Input: dimensioned drawing with shaded views. Units: mm. Origin: part minimum x, y, z. A direction names the side the tool comes from. Give positions to 0.01 mm unless a question says otherwise; leave off trailing zeros. Loops run counter-clockwise (first coordinate to the right, second up) from the corner with the lowest first, then second, coordinate; pieces in that order, holes last. Notation, with made-up numbers: M 53,10.5 L 93,10.5 A21 ccw 93,41.5 Z; hole C 37.5,69.25 d10. An arc over 180 degrees is marked long. Use CSV: the item, a comma, the result in double quotes. Start each with the question number.
Q1. Pull-direction query (X, two-part tool) for the marked faces 3, 4 and 5; classes: released by +X, released by -X, zero draft, split by the parting line, or undercut.
Q2. Section D-D, the plane z = 19. Output: boundary loops of the cut face in (x, y), plus the area to 3 significant figures.
Q3. Reachability of the marked faces 1 and 2 from +Z, -Z, +X, -X, +Y, -Y: full face, straight path, thin tool, end or side. Return the list, or none.
Q4. Material intervals for line 1 along X through (y, z) = (5.75, 48.5) (1 decimal); line 2 along X through (y, z) = (0.75, 27.5); line 3 along Z through (x, y) = (49.75, 4), sorted ascending.
Q5. Section A-A, the plane z = 27.25. Output: boundary loops of the cut face in (x, y), plus the area to 3 significant figures.
Q6. Section B-B, the plane x = 27.25. Output: boundary loops of the cut face in (y, z).
Q7. Pin query (flat end, axial travel): pin 1 (5 mm diameter, centred on x = 11, z = 34, fed in from +Y); pin 2 (4 mm diameter, centred on y = 2, z = 42.5, fed in from -X); pin 3 (4.5 mm diameter, centred on x = 9.05, z = 40.48, fed in from +Y); pin 4 (2 mm diameter, centred on y = 2, z = 10.5, fed in from -X). Return the tip coordinate at first contact, or that it passes through.
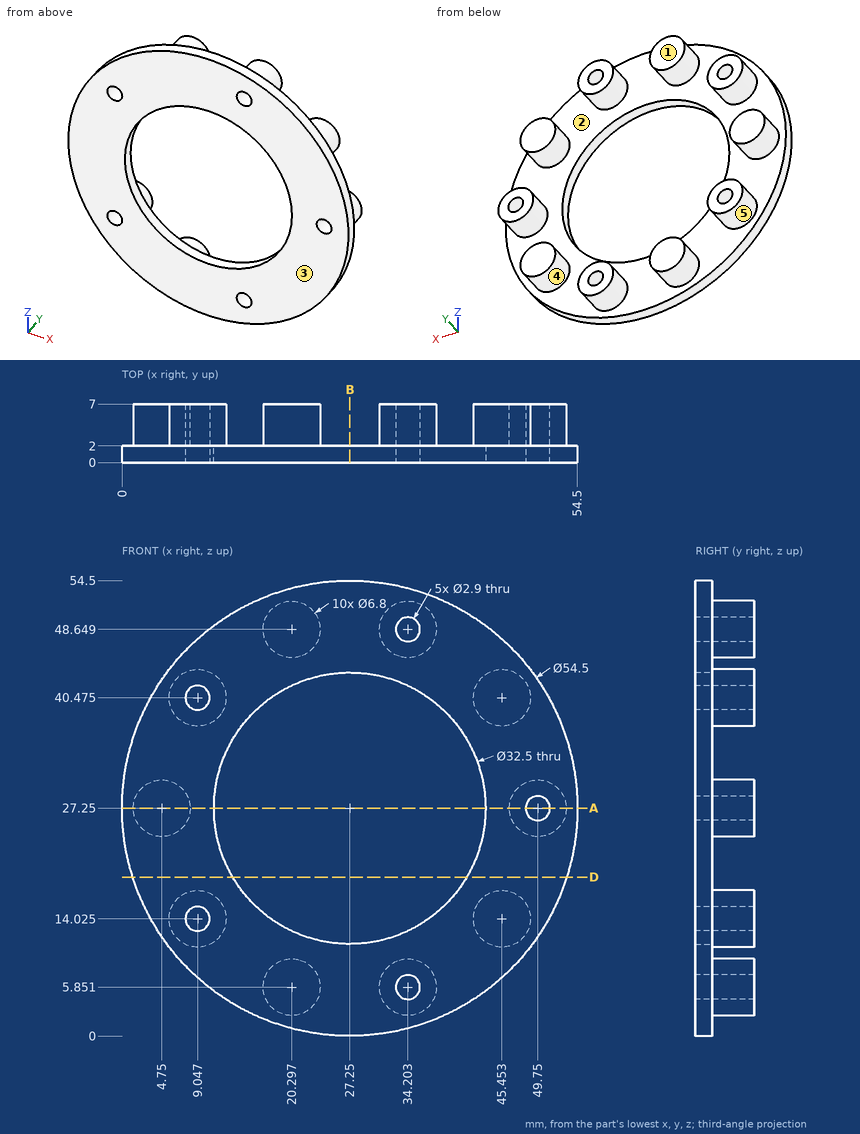
A:
1,face 3,"zero draft"
1,face 4,"undercut"
1,face 5,"undercut"
2,outline,"M 1.28,0 L 13.25,0 L 13.25,2 L 1.28,2 Z; M 41.25,0 L 53.22,0 L 53.22,2 L 41.25,2 Z"
2,area,"47.9 mm^2"
3,face 1,"+Z, -Z, +X, -X, +Y"
3,face 2,"+Y"
4,line 1,"16.9 to 23.7, 30.8 to 32.8, 35.6 to 37.6"
4,line 2,"0 to 11, 43.5 to 48.32, 51.18 to 54.5"
4,line 3,"23.85 to 25.8, 28.7 to 30.65"
5,outline,"M 0,0 L 11,0 L 11,2 L 8.15,2 L 8.15,7 L 1.35,7 L 1.35,2 L 0,2 Z; M 43.5,0 L 48.3,0 L 48.3,7 L 46.35,7 L 46.35,2 L 43.5,2 Z; M 51.2,0 L 54.5,0 L 54.5,2 L 53.15,2 L 53.15,7 L 51.2,7 Z"
5,area,"91.7 mm^2"
6,outline,"M 0,0 L 2,0 L 2,11 L 0,11 Z; M 0,43.5 L 2,43.5 L 2,54.5 L 0,54.5 Z"
7,pin 1,"y = 2"
7,pin 2,"x = 3.44"
7,pin 3,"y = 7"
7,pin 4,"x = 5.01"
